from build123d import *

# Parameters (mm, degrees)
ESQUISSE1_R        = 5
ESQUISSE1_R_2      = 4.5
BOSS_EXTRU_1_DEPTH = 9
ESQUISSE2_R        = 6
ESQUISSE2_R_2      = 5
ESQUISSE2_R_3      = 4.5
BOSS_EXTRU_2_DEPTH = 1.5
ESQUISSE3_R        = 6
ESQUISSE3_R_2      = 5
BOSS_EXTRU_3_DEPTH = 2.5


with BuildPart() as part:
    # Esquisse1 → Boss.-Extru.1 (new body)
    with BuildSketch(Plane(origin=(0, 0, 0), x_dir=(1, 0, 0), z_dir=(0, 1, 0))):
        with Locations(Location((0, 0, 0), (0, 0, 270))):
            Circle(ESQUISSE1_R)
        with Locations(Location((0, 0, 0), (0, 0, 270))):
            Circle(ESQUISSE1_R_2, mode=Mode.SUBTRACT)
    extrude(amount=BOSS_EXTRU_1_DEPTH)

    # Esquisse2 → Boss.-Extru.2 (add)
    # profile 1 of 2: a face of its own
    with BuildSketch(Plane(origin=(0, 9, 0), x_dir=(1, 0, 0), z_dir=(0, 1, 0))):
        with Locations(Location((0, 0, 0), (0, 0, 270))):
            Circle(ESQUISSE2_R)
        with Locations(Location((0, 0, 0), (0, 0, 270))):
            Circle(ESQUISSE2_R_2, mode=Mode.SUBTRACT)
    # profile 2 of 2: a face of its own
    with BuildSketch(Plane(origin=(0, 9, 0), x_dir=(1, 0, 0), z_dir=(0, 1, 0))):
        with Locations(Location((0, 0, 0), (0, 0, 270))):
            Circle(ESQUISSE2_R_2)
        with Locations(Location((0, 0, 0), (0, 0, 270))):
            Circle(ESQUISSE2_R_3, mode=Mode.SUBTRACT)
    extrude(amount=BOSS_EXTRU_2_DEPTH)

    # Esquisse3 → Boss.-Extru.3 (add)
    with BuildSketch(Plane(origin=(0, 10.5, 0), x_dir=(1, 0, 0), z_dir=(0, 1, 0))):
        with Locations(Location((0, 0, 0), (0, 0, 270))):
            Circle(ESQUISSE3_R)
        with Locations(Location((0, 0, 0), (0, 0, 270))):
            Circle(ESQUISSE3_R_2, mode=Mode.SUBTRACT)
    extrude(amount=BOSS_EXTRU_3_DEPTH)


solid = part.part
The model under review builds one solid part; all positions refer to its coordinate system, in mm. A direction names the side the tool comes from. Give positions to 0.01 mm unless a question says otherwise; leave off trailing zeros. Order: outer loops, then holes, each group sorted by start corner. A loop starts at its lowest first (then second) coordinate and runs counter-clockwise, first axis right, second up. Notation, with made-up numbers: M 43.5,14.5 L 82.5,14.5 A24 cw 82.5,28.5 Z; hole C 48.25,-31 d8. An arc over 180 degrees is marked long. Use one line per item in the form item = value. Start each with the question number.
Item 1: For faces 4 (the cylindrical face through (-4.88, 4.44, -1.08)), 5 (the flat face through (4, 13, -4)), 6 (the cylindrical face through (-4.88, 11.73, -1.08)), list the 3-axis set-ups (+Z, -Z, +X, -X, +Y, -Y) from which the entire face can be reached by the end or side of a thin tool; tool diameter is ignored.
Item 2: To check wall thickness, follow line 1 along X through (y, z) = (11.65, 0); line 2 along X through (y, z) = (6.75, 0); line 3 along Z through (x, y) = (2, 10). State the ranges of each line that lie inside material, in increasing order. Write a range as from..to.
Item 3: Insertion check: pin 1 Ø5 at (x, y) = (-4.5, 4) entering from +Z; pin 2 Ø6 at (x, z) = (0, 0) entering from +Y; pin 3 Ø5 at (y, z) = (7, 3) entering from -X. Each pin has a flat end and moves straight along its axis. Give the tip position at first contact, or say it passes through.
Item 4: We need section A-A on x = 0. Give the boundary of the cut face in (y, z).
Item 5: We need section D-D on y = 12. Give the boundary of the cut face in (x, z).
Item 6: The part is to be moulded in two halves that separate along Z. For faces 1 (the cylindrical face through (1.802, 10.972, 5.723)), 2 (the cylindrical face through (1.352, 5.176, 4.292)), 3 (the flat face through (4, 9, -4)), say which applies: pulls with the +Z half, pulls with the -Z half, needs draft (parallel to the pull), parting line crosses it, or undercut.
Item 7: We need section B-B on z = 0. Give the boundary of the cut face in (x, y).
Item 8: We need section C-C on y = 7.25. Give the boundary of the cut face in (x, z).
Completed:
q1.face_4 = -Y
q1.face_5 = +Z, -Z, +X, -X, +Y
q1.face_6 = +Y
q2.line_1 = -6..-5, 5..6
q2.line_2 = -5..-4.5, 4.5..5
q2.line_3 = -5.66..-4.03, 4.03..5.66
q3.pin_1 = 4.58
q3.pin_2 = through
q3.pin_3 = -5.81
q4.outline = M 0,-5 L 9,-5 L 9,-6 L 13,-6 L 13,-5 L 10.5,-5 L 10.5,-4.5 L 0,-4.5 Z; M 0,4.5 L 10.5,4.5 L 10.5,5 L 13,5 L 13,6 L 9,6 L 9,5 L 0,5 Z
q5.outline = C 0,0 d12; hole C 0,0 d10
q6.face_1 = parting line crosses it
q6.face_2 = undercut
q6.face_3 = needs draft
q7.outline = M -6,9 L -5,9 L -5,0 L -4.5,0 L -4.5,10.5 L -5,10.5 L -5,13 L -6,13 Z; M 4.5,0 L 5,0 L 5,9 L 6,9 L 6,13 L 5,13 L 5,10.5 L 4.5,10.5 Z
q8.outline = C 0,0 d10; hole C 0,0 d9
